Work out the finished part from the listing and answer in its coordinate system (mm). A direction names the side the tool comes from. Coordinates: 2 decimals unless noted, no trailing zeros. Order: outer loops, then holes, each group sorted by start corner. A loop starts at its lowest first (then second) coordinate and runs counter-clockwise, first axis right, second up. Notation, with made-up numbers: (67.5, -2) -> (99.5, -2) arc R36 ccw to (99.5, 36) -> close; hole circle Ø1 at (-30.75, 54). An arc over 180 degrees is marked (long way). Write item = value, one per line. Start each with the question number.
Q1. For a pull along X with two mould halves and no side action, classify faces 1 (the flat face through (2, -5, -12)), 2 (the cylindrical face through (1.172, 8.923, 10.989)), 3 (the cylindrical face through (-1.08, -4.88, 0.17)) as +X half, -X half, draft (parallel to the pull), parting line (faces both ways), or undercut.
Q2. The part is cut by section C-C, the plane z = -4. Determine the outline of the cut face in (x, y), plus the area to 3 significant figures.
Q3. Straight lines are drawn through the part: L1, parallel to Y at x = 0, z = 4; L2, parallel to Z at x = -2.25, y = -7; L3, parallel to Y at x = 1.5, z = 3.5. For each, find the intervals that lie inside material, in ascending order. Write a range as from..to.
Q4. Which of the six approach directions +Z, -Z, +X, -X, +Y, -Y give full straight-line access (tool end or side, diameter ignored) to faces 4 (the cylindrical face through (1.515, -6.824, -1.151)), 5 (the flat face through (4, -4, 12))?
Q5. Flat-ended cylindrical pins translate along their axes: pin 1 (1 mm diameter, centred on y = 5, z = 1, fed in from +X); pin 2 (1 mm diameter, centred on y = -0.5, z = 7.5, fed in from -X); pin 3 (2 mm diameter, centred on y = -3, z = -3, fed in from +X). Find the tip coordinate at first contact, or state that the pin passes through.
Q6. The part is cut by section A-A, the plane y = 0. Determine the outline of the cut face in (x, z), plus the area to 3 significant figures.
```python
from build123d import *

# Parameters (mm, degrees)
F2_R          = 5
F3_DEPTH      = 12.001
F3_DEPTH_BACK = 25
F4_SIZE       = 0.2
F5_R          = 0.2


with BuildPart() as f1:
    # F0 (on Front) → F1 (revolve)
    with BuildSketch(Plane.XZ):
        Polygon((0, -12), (0, 12), (-9, 12), (-9, 10), (-6.99, 10), (-6.99, -12), align=None)
    revolve(axis=Axis((0, 0, -0.6447483601), (0, 0, -1)))

    # F2 (on Top) → F3 (cut, two sides)
    with BuildSketch(Plane.XY) as f3_sk:
        Circle(F2_R)
    extrude(amount=-F3_DEPTH, mode=Mode.SUBTRACT)
    extrude(f3_sk.sketch, amount=F3_DEPTH_BACK, mode=Mode.SUBTRACT)

    # F4
    f4_edges = [f1.edges().sort_by_distance(p)[0] for p in [
        (-5, 0, -12),
        (6.99, 0, -12),
        (9, 0, 10),
        (9, 0, 12),
        (-5, 0, 12),
    ]]
    chamfer(f4_edges, length=F4_SIZE)

    # F5
    f5_edges = [f1.edges().sort_by_distance(p)[0] for p in [
        (6.99, 0, 10),
    ]]
    fillet(f5_edges, radius=F5_R)


solid = f1.part
```
Model answer:
q1.face_1 = draft
q1.face_2 = parting line
q1.face_3 = undercut
q2.outline = circle Ø13.98 at (0, 0); hole circle Ø10 at (0, 0)
q2.area = 75.0 mm2
q3.L1 = -6.99..-5, 5..6.99
q3.L2 = 10..12
q3.L3 = -6.83..-4.77, 4.77..6.83
q4.face_4 = -Z
q4.face_5 = +Z, +X, -X, +Y, -Y
q5.pin_1 = 5.35
q5.pin_2 = -6.99
q5.pin_3 = 6.7
q6.outline = (-9, 10.2) -> (-8.8, 10) -> (-7.19, 10) arc R0.2 cw to (-6.99, 9.8) -> (-6.99, -11.8) -> (-6.79, -12) -> (-5.2, -12) -> (-5, -11.8) -> (-5, 11.8) -> (-5.2, 12) -> (-8.8, 12) -> (-9, 11.8) -> close; (5, -11.8) -> (5.2, -12) -> (6.79, -12) -> (6.99, -11.8) -> (6.99, 9.8) arc R0.2 cw to (7.19, 10) -> (8.8, 10) -> (9, 10.2) -> (9, 11.8) -> (8.8, 12) -> (5.2, 12) -> (5, 11.8) -> close
q6.area = 103 mm2
